Source: CAD feature listing. Evaluate the final solid. Frame: model axes, mm. A direction names the side the tool comes from. Round coordinates to 2 decimals unless told otherwise and drop trailing zeros. Loops run counter-clockwise (first coordinate to the right, second up) from the corner with the lowest first, then second, coordinate; pieces in that order, holes last. Notation, with made-up numbers: (82.25, 85.25) -> (119.25, 85.25) arc R7 cw to (119.25, 89.25) -> close; hole circle Ø7 at (-39, 32.25). An arc over 180 degrees is marked (long way). Write item = value, one per line.
from build123d import *

# Parameters (mm, degrees)
BOSS_EXTRUDE1_DEPTH = 7.9375
BOSS_EXTRUDE2_DEPTH = 1.5875


with BuildPart() as part:
    # Sketch1 → Boss-Extrude1 (new, symmetric)
    with BuildSketch(Plane.XY):
        with BuildLine():
            Line((28.2575, -12.7), (28.2575, -3.33375))
            ThreePointArc((28.2575, -3.33375), (27.513551224, -1.537698776), (25.7175, -0.79375))
            Line((25.7175, -0.79375), (6.594808295, -0.79375))
            Line((6.594808295, -0.79375), (6.594808295, 0.79375))
            Line((6.594808295, 0.79375), (25.7175, 0.79375))
            ThreePointArc((25.7175, 0.79375), (27.513551224, 1.537698776), (28.2575, 3.33375))
            Line((28.2575, 3.33375), (28.2575, 12.7))
            Line((28.2575, 12.7), (17.4625, 12.7))
            ThreePointArc((17.4625, 12.7), (16.411440521, 12.927669147), (15.54880137, 13.569863014))
            ThreePointArc((15.54880137, 13.569863014), (0.91366194, 20.617265292), (-14.2875, 14.892070037))
            Line((-14.2875, 14.892070037), (-25.033653846, 4.582175396))
            ThreePointArc((-25.033653846, 4.582175396), (-26.9875, 0), (-25.033653846, -4.582175396))
            Line((-25.033653846, -4.582175396), (-14.2875, -14.892070037))
            ThreePointArc((-14.2875, -14.892070037), (0.91366194, -20.617265292), (15.54880137, -13.569863014))
            ThreePointArc((15.54880137, -13.569863014), (16.411440521, -12.927669147), (17.4625, -12.7))
            Line((17.4625, -12.7), (28.2575, -12.7))
        make_face()
    extrude(amount=BOSS_EXTRUDE1_DEPTH, both=True)

    # Sketch2 → Cut-Revolve1 (revolve, cut)
    with BuildSketch(Plane(origin=(0, 0, 0), x_dir=(0, 0, -1), z_dir=(1, 0, 0))):
        Polygon((5.0038, 16.256), (-5.0038, 16.256), (-6.381996671, 11.1125), (-17.041212854, 11.1125), (-17.041212854, 0), (17.041212854, 0), (17.041212854, 11.1125), (6.381996671, 11.1125), align=None)
    revolve(axis=Axis((0, 0, -17.041212854), (0, 0, -1)), mode=Mode.SUBTRACT)

    # Sketch3 → Revolve1 (revolve)
    with BuildSketch(Plane.XY):
        Polygon((22.86, 12.7), (27.6225, 12.7), (27.6225, 13.530402551), (25.834540931, 23.283333333), (25.00413838, 23.283333333), (25.00413838, 27.813), (24.24213838, 28.575), (22.86, 28.575), (22.86, 23.283333333), (22.86, 17.991666667), align=None)
    revolve(axis=Axis((22.86, 28.575, 0), (0, 1, 0)))

    # Sketch4 → Boss-Extrude2 (add, symmetric)
    with BuildSketch(Plane.XY):
        with BuildLine():
            Line((25.261436698, 22.452930783), (26.351802053, 24.0328217))
            ThreePointArc((26.351802053, 24.0328217), (27.98426331, 25.088440013), (29.885022603, 24.680550456))
            Line((29.885022603, 24.680550456), (31.474518222, 23.583556394))
            ThreePointArc((31.474518222, 23.583556394), (32.530136536, 21.951095136), (32.122246979, 20.050335843))
            Line((32.122246979, 20.050335843), (27.049395767, 12.7))
            Line((27.049395767, 12.7), (25.261436698, 22.452930783))
        make_face()
        with BuildLine():
            Line((20.458563302, 22.452930783), (18.670604233, 12.7))
            Line((18.670604233, 12.7), (13.597753021, 20.050335843))
            ThreePointArc((13.597753021, 20.050335843), (13.189863464, 21.951095136), (14.245481778, 23.583556394))
            Line((14.245481778, 23.583556394), (15.834977397, 24.680550456))
            ThreePointArc((15.834977397, 24.680550456), (17.73573669, 25.088440013), (19.368197947, 24.0328217))
            Line((19.368197947, 24.0328217), (20.458563302, 22.452930783))
        make_face()
    extrude(amount=BOSS_EXTRUDE2_DEPTH, both=True)


solid = part.part
1. Section query B-B (x = 22.86). Return the cut outline in (y, z) (1 decimal), then the cut area to 3 significant figures.
Evaluation:
outline = (-12.7, -7.9) -> (-0.8, -7.9) -> (-0.8, 7.9) -> (-12.7, 7.9) -> close; (0.8, -7.9) -> (12.7, -7.9) -> (12.7, -4.8) -> (13.5, -4.8) -> (23.3, -3) -> (23.3, -2.1) -> (27.8, -2.1) -> (28.6, -1.4) -> (28.6, 1.4) -> (27.8, 2.1) -> (23.3, 2.1) -> (23.3, 3) -> (13.5, 4.8) -> (12.7, 4.8) -> (12.7, 7.9) -> (0.8, 7.9) -> close
area = 484 mm²
2. Contact query for flat-ended pins moving along their axis: pin 1 Ø2 at (x, y) = (17, 19.5) entering from +Z; pin 2 Ø8 at (x, z) = (10, -3.5) entering from +Y; pin 3 Ø1.5 at (y, z) = (13.5, 5.5) entering from -X. Output: stop coordinate, or through.
Evaluation:
pin_1 = 1.59
pin_2 = 22.8
pin_3 = -16.52
3. Mould query, pull axis Y, two halves, no side actions, for faces 5 (the face through (-26.987, 0.072, 0.111)), 6 (the face through (21.158, 25.58, 1.305)), 7 (the face through (27.533, -1.558, 0.111)). Classes: released by +Y, released by -Y, zero draft, split by the parting line, or undercut.
Evaluation:
face_5 = split by the parting line
face_6 = zero draft
face_7 = undercut
4. Set-up query: faces 1 (the face through (17.708, 25.093, 0.022)), 2 (the face through (20, -0.794, 0)), 3 (the face through (18.1, 13.1, -0.2)), 4 (the face through (17, 21, -1.588)). Return all of +Z, -Z, +X, -X, +Y, -Y with unobstructed straight access to the full face (end or side cutting, diameter ignored); none if empty.
Evaluation:
face_1 = +Z, -Z, +Y
face_2 = +Z, -Z, +X
face_3 = none
face_4 = -Z, +Y
5. Section query C-C (y = 0). Return the cut outline in (x, z).
Evaluation:
outline = (-26.99, -7.94) -> (-11.11, -7.94) -> (-11.11, -6.38) -> (-16.26, -5) -> (-16.26, 5) -> (-11.11, 6.38) -> (-11.11, 7.94) -> (-26.99, 7.94) -> close
6. Line query: probe 1 along Y at (x, z) = (0, 7.15); probe 2 along Y at (x, z) = (21, 6.5); probe 3 along Y at (x, z) = (17.5, 0.25). Output: solid intervals per line, ascending. Write a range as from..to.
Evaluation:
probe_1 = -20.64..-11.11, 11.11..20.64
probe_2 = -12.7..-0.79, 0.79..12.7
probe_3 = -12.7..-0.79, 0.79..12.7, 14.4..25.12
7. Section query A-A (y = 19). Return the cut outline in (x, z), then the cut area to 3 significant figures.
Evaluation:
outline = (-8.06, -7.94) -> (8.06, -7.94) -> (8.06, 7.94) -> (-8.06, 7.94) -> close; (14.32, -1.59) -> (19.45, -1.59) arc R3.76 ccw to (26.27, -1.59) -> (31.4, -1.59) -> (31.4, 1.59) -> (26.27, 1.59) arc R3.76 ccw to (19.45, 1.59) -> (14.32, 1.59) -> close
area = 331 mm²
